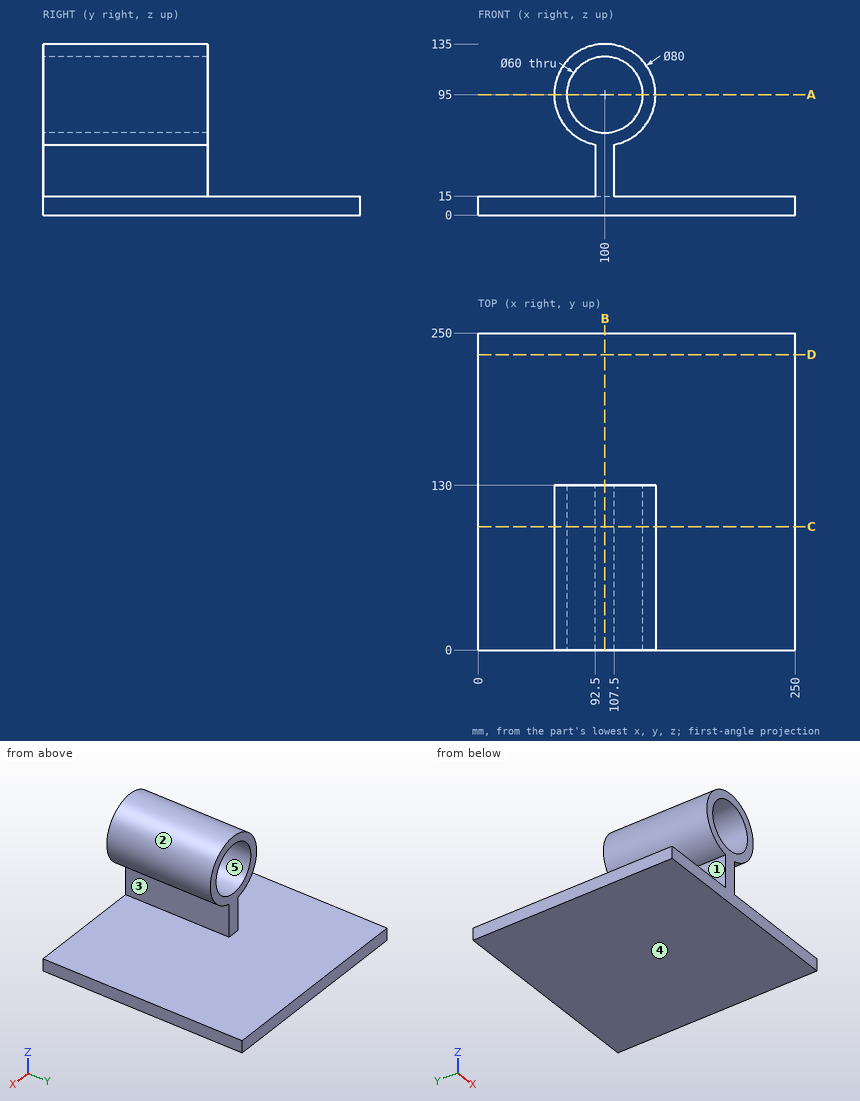
Verification items for this drawing (mm, ordinates from the low corner). A direction names the side the tool comes from. Give positions to 0.01 mm unless a question says otherwise; leave off trailing zeros. Write each loop counter-clockwise with the first axis right and the second up, starting at its lowest first coordinate (ties: lowest second). Pieces come first, ordered by that corner, then holes. Notation, with made-up numbers: (75.25, 85.5) -> (103.25, 85.5) arc R19 cw to (103.25, 100.5) -> close; hole circle Ø5 at (16.25, -13.5). An arc over 180 degrees is marked (long way). Use one line per item in the form item = value.
Item 1: Sectioned sample at D-D on y = 233. Enter the section's corners in (x, z), plus the area to 3 significant figures.
Results list:
outline = (0, 0) -> (250, 0) -> (250, 15) -> (0, 15) -> close
area = 3,750 mm2
Item 2: Sectioned sample at C-C on y = 97.5. Enter the section's corners in (x, z), plus the area to 3 significant figures.
Results list:
outline = (0, 0) -> (250, 0) -> (250, 15) -> (107.5, 15) -> (107.5, 55.71) arc R40 ccw (long way) to (92.5, 55.71) -> (92.5, 15) -> (0, 15) -> close; hole circle Ø60 at (100, 95)
area = 6,550 mm2
Item 3: Sectioned sample at B-B on x = 100. Enter the section's corners in (y, z).
Results list:
outline = (0, 0) -> (250, 0) -> (250, 15) -> (130, 15) -> (130, 65) -> (0, 65) -> close; (0, 125) -> (130, 125) -> (130, 135) -> (0, 135) -> close
Item 4: Mould release check, pull along Z, two halves, no side actions. Record for the marked faces 4 and 5: released by +Z, released by -Z, zero draft, split by the parting line, or undercut.
Results list:
face_4 = released by -Z
face_5 = undercut
Item 5: Scan lines: line 1 (X direction, y = 41, z = 96); line 2 (Z direction, x = 100, y = 45); line 3 (X direction, y = 47, z = 31). Record each from-to range of solid material in increasing order.
Results list:
line_1 = 60.01 to 70.02, 129.98 to 139.99
line_2 = 0 to 65, 125 to 135
line_3 = 92.5 to 107.5
Item 6: Access from +Z, -Z, +X, -X, +Y, -Y to the whole of each face (thin tool, end or side, straight path). Record for the marked faces 1, 2 and 3.
Results list:
face_1 = -X, +Y, -Y
face_2 = +Y, -Y
face_3 = +X, +Y, -Y
Item 7: Depth check by flat-ended pin: pin 1 Ø20.5 at (y, z) = (32.5, 43) entering from -X; pin 2 Ø1.5 at (y, z) = (74.5, 78) entering from +X; pin 3 Ø3 at (y, z) = (130.5, 66) entering from +X. Enter the tip coordinate at first touch or a pass-through.
Results list:
pin_1 = 92.5
pin_2 = 136.55
pin_3 = 128.97
Item 8: Sectioned sample at A-A on z = 95. Enter the section's corners in (x, y), plus the area to 3 significant figures.
Results list:
outline = (60, 0) -> (70, 0) -> (70, 130) -> (60, 130) -> close; (130, 0) -> (140, 0) -> (140, 130) -> (130, 130) -> close
area = 2,600 mm2
